```python
from build123d import *

# Parameters (mm, degrees)
SKETCH1_R             = 40
BOSS_EXTRUDE1_DEPTH   = 9
SKETCH2_R             = 38
SKETCH2_R_2           = 33
BOSS_EXTRUDE2_DEPTH   = 9
F_8_0MM_DOWEL_HOLE1_D = 8


with BuildPart() as part:
    # Sketch1 → Boss-Extrude1 (new body)
    with BuildSketch(Plane(origin=(0, 0, 0), x_dir=(1, 0, 0), z_dir=(0, 1, 0))):
        with Locations(Location((0, 0, 0), (0, 0, 270))):
            Circle(SKETCH1_R)
    extrude(amount=BOSS_EXTRUDE1_DEPTH)

    # Sketch2 → Boss-Extrude2 (add)
    with BuildSketch(Plane.XZ):
        with Locations(Location((0, 0, 0), (0, 0, 90))):
            Circle(SKETCH2_R)
        with Locations(Location((0, 0, 0), (0, 0, 270))):
            Circle(SKETCH2_R_2, mode=Mode.SUBTRACT)
    extrude(amount=BOSS_EXTRUDE2_DEPTH)

    # Ø8.0mm Dowel Hole1 (through all)
    with Locations(Plane(origin=(0, 0, 0), x_dir=(-1, 0, 0), z_dir=(0, -1, 0))):
        with Locations((-28, 0), (28, 0)):
            Hole(F_8_0MM_DOWEL_HOLE1_D / 2)


solid = part.part
```
Geometry: final body of the model. Coordinates: model frame, mm. A direction names the side the tool comes from. Coordinates: 2 decimals unless noted, no trailing zeros. Loops run counter-clockwise (first coordinate to the right, second up) from the corner with the lowest first, then second, coordinate; pieces in that order, holes last. Notation, with made-up numbers: (-9, 65.25) -> (31, 65.25) arc R27 cw to (31, 104.25) -> close; hole circle Ø8 at (-8, 51.25). An arc over 180 degrees is marked (long way). Use a Markdown table: item, result. Add a question column.
(1) Access query for faces 4 (the cylindrical face through (24.8, 4.6, 2.4)), 5 (the cylindrical face through (23.122, -4.437, -30.156)). Directions: +Z, -Z, +X, -X, +Y, -Y. A direction counts if a zero-diameter tool reaches every point of the face in a straight line with its end or side. Return the directions, or none.
(2) Mould query, pull axis X, two halves, no side actions, for faces 1 (the flat face through (1, 9, -1)), 2 (the cylindrical face through (-39.05, 4.44, -8.67)), 3 (the flat face through (0, 0, 0)). Classes: pulls with the +X half, pulls with the -X half, needs draft (parallel to the pull), parting line crosses it, or undercut.
(3) Line query: line 1 along Y through (x, z) = (-2.5, -28.5); line 2 along Z through (x, y) = (29.5, -8); line 3 along X through (y, z) = (6.25, 3). Output: solid intervals per line, ascending.
(4) Section query B-B, the plane x = 28. Return loops of the section in (y, z).
(5) Section query A-A, the plane z = 0. Return loops of the section in (x, y).
(6) Section query D-D, the plane x = 0. Return loops of the section in (y, z), plus the area to 3 significant figures.
(7) Section query C-C, the plane y = 2.5. Return loops of the section in (x, z).
(8) Pin query (flat end, axial travel): pin 1 Ø6 at (y, z) = (-2, -7.5) entering from -X; pin 2 Ø3 at (y, z) = (-4, -6) entering from +X; pin 3 Ø4 at (y, z) = (2.5, 0.5) entering from +X; pin 4 Ø6.5 at (x, z) = (-28, 0) entering from -Y. Return the tip coordinate at first contact, or that it passes through.
Answer:
| question | item | result |
|---|---|---|
| 1 | face 4 | +Y, -Y |
| 1 | face 5 | -Y |
| 2 | face 1 | needs draft |
| 2 | face 2 | parting line crosses it |
| 2 | face 3 | undercut |
| 3 | line 1 | y = 0 to 9 |
| 3 | line 2 | z = -23.95 to -14.79, 14.79 to 23.95 |
| 3 | line 3 | x = -39.89 to -30.65, -25.35 to 25.35, 30.65 to 39.89 |
| 4 | outline | (-9, -25.69) -> (0, -25.69) -> (0, -28.57) -> (9, -28.57) -> (9, -4) -> (0, -4) -> (0, -17.46) -> (-9, -17.46) -> close; (-9, 17.46) -> (0, 17.46) -> (0, 4) -> (9, 4) -> (9, 28.57) -> (0, 28.57) -> (0, 25.69) -> (-9, 25.69) -> close |
| 5 | outline | (-40, 0) -> (-38, 0) -> (-38, -9) -> (-33, -9) -> (-33, 0) -> (-32, 0) -> (-32, 9) -> (-40, 9) -> close; (-24, 0) -> (24, 0) -> (24, 9) -> (-24, 9) -> close; (32, 0) -> (33, 0) -> (33, -9) -> (38, -9) -> (38, 0) -> (40, 0) -> (40, 9) -> (32, 9) -> close |
| 6 | outline | (-9, -38) -> (0, -38) -> (0, -40) -> (9, -40) -> (9, 40) -> (0, 40) -> (0, 38) -> (-9, 38) -> (-9, 33) -> (0, 33) -> (0, -33) -> (-9, -33) -> close |
| 6 | area | 810 mm^2 |
| 7 | outline | circle Ø80 at (0, 0); hole circle Ø8 at (-28, 0); hole circle Ø8 at (28, 0) |
| 8 | pin 1 | stops at x = -39.65 |
| 8 | pin 2 | stops at x = 37.73 |
| 8 | pin 3 | stops at x = 40 |
| 8 | pin 4 | passes through |
